from build123d import *

# Parameters (mm, degrees)
SWEEP_THIN1_PROFILE_R   = 6
SWEEP_THIN1_PROFILE_R_2 = 5


with BuildPart() as part:
    # Sweep-Thin1: sweep along a path in Sketch1
    with BuildLine(Plane.XY) as sweep_thin1_path:
        Line((-25, 45), (-10, 45))
        ThreePointArc((-10, 45), (-2.928932188, 42.071067812), (0, 35))
        Line((0, 35), (0, 10))
        ThreePointArc((0, 10), (2.928932188, 2.928932188), (10, 0))
        Line((10, 0), (25, 0))
    # Sweep-Thin1 profile (on start of the path) → Sweep-Thin1 (sweep)
    with BuildSketch(Plane(origin=(-25, 45, 0), x_dir=(0, 0, 1), z_dir=(1, 0, 0))):
        Circle(SWEEP_THIN1_PROFILE_R)
        Circle(SWEEP_THIN1_PROFILE_R_2, mode=Mode.SUBTRACT)
    sweep(path=sweep_thin1_path.line)


solid = part.part
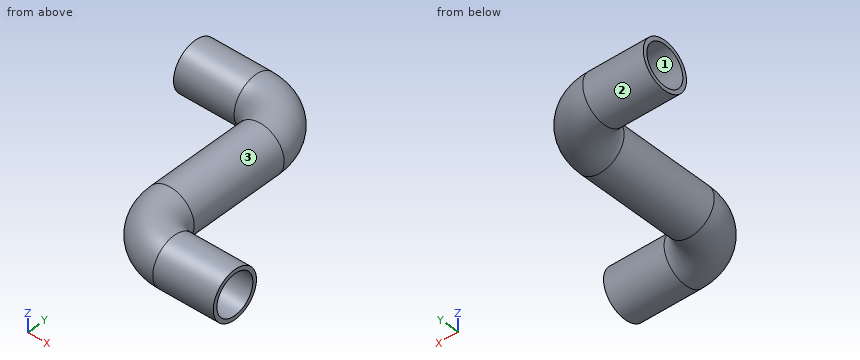
CAD build for the part. Positions are in the model's coordinates, mm. Face numbers are marked on the shaded views. Round coordinates to 2 decimals unless told otherwise and drop trailing zeros. Loops run counter-clockwise (first coordinate to the right, second up) from the corner with the lowest first, then second, coordinate; pieces in that order, holes last.
(1) Cut at B-B (x = 18.5). Give the cut face in (y, z), plus the area to 3 significant figures.
(2) Wall check: line 1 along Z through (x, y) = (16.75, 0); line 2 along Z through (x, y) = (-4, 27.5). Give the ranges that are in metal, low to high.
(3) Cut at A-A (z = 0). Give the cut face in (x, y), plus the area to 3 significant figures.
(4) Two-plate mould, pull along Y, no slides. Class the marked faces 1, 2 and 3: +Y half, -Y half, draft (parallel to the pull), parting line (faces both ways), or undercut.
(5) Drop flat-ended pins along their axis: pin 1 (5 mm diameter, centred on y = 12.5, z = 4, fed in from +X); pin 2 (4 mm diameter, centred on y = 7, z = 3, fed in from -X); pin 3 (1 mm diameter, centred on y = 40.5, z = -1, fed in from -X); pin 4 (2 mm diameter, centred on x = -15, z = 1.5, fed in from -Y). Give the stop position or say it passes through.
Findings below:
1. outline: circle Ø12 at (0, 0); hole circle Ø10 at (0, 0)
1. area: 34.6 mm2
2. line 1: z = -6 to -5, 5 to 6
2. line 2: z = -4.47 to -3, 3 to 4.47
3. outline: (-25, 39) - (-10, 39) arc R4 cw to (-6, 35) - (-6, 10) arc R16 ccw to (10, -6) - (25, -6) - (25, -5) - (10, -5) arc R15 cw to (-5, 10) - (-5, 35) arc R5 ccw to (-10, 40) - (-25, 40) - close; (-25, 50) - (-10, 50) arc R15 cw to (5, 35) - (5, 10) arc R5 ccw to (10, 5) - (25, 5) - (25, 6) - (10, 6) arc R4 cw to (6, 10) - (6, 35) arc R16 ccw to (-10, 51) - (-25, 51) - close
3. area: 173 mm2
4. face 1: undercut
4. face 2: parting line
4. face 3: draft
5. pin 1: stops at x = 5.81
5. pin 2: stops at x = -5.74
5. pin 3: stops at x = -25
5. pin 4: stops at y = 39.02
